For this review, use the dimensioned drawing (mm, ordinates from the lowest corner) and the shaded views. A direction names the side the tool comes from. Give positions to 0.01 mm unless a question says otherwise; leave off trailing zeros. Loops run counter-clockwise (first coordinate to the right, second up) from the corner with the lowest first, then second, coordinate; pieces in that order, holes last. Notation, with made-up numbers: (51.25, -22.5) - (106.25, -22.5) arc R28 cw to (106.25, -1.5) - close; hole circle Ø5 at (79, -31.5). An arc over 180 degrees is marked (long way). Write each question's results on one line, items separated by ' | '.
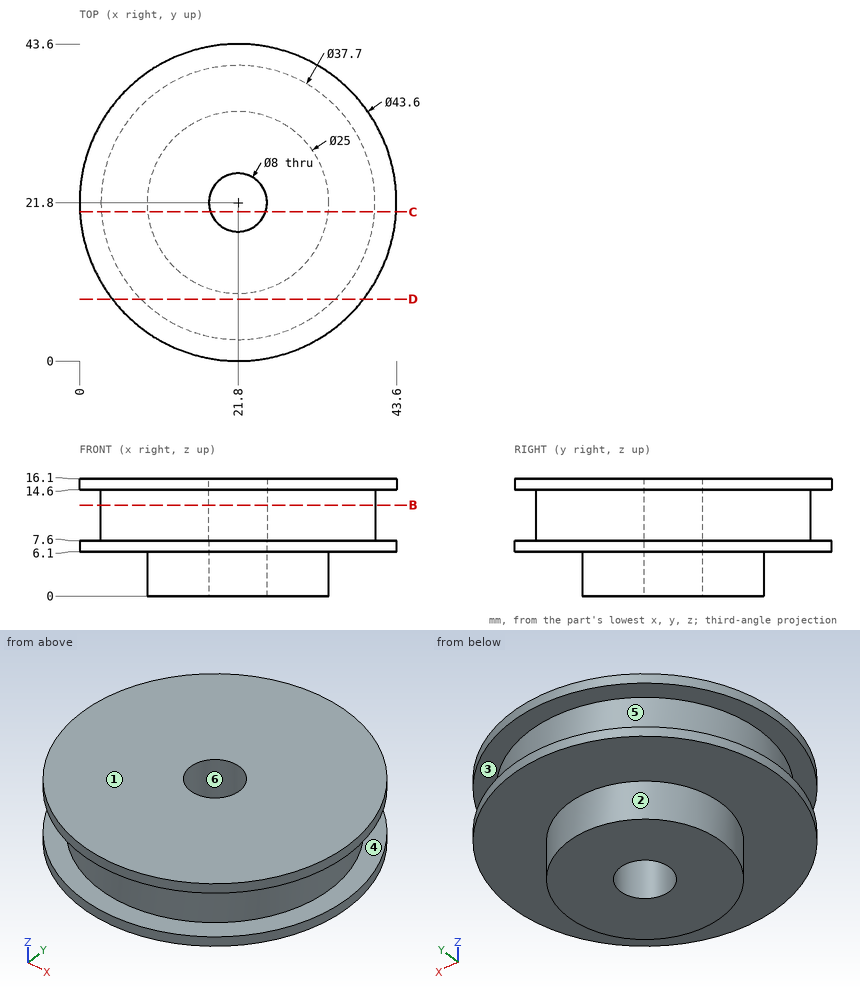
Item 1: We need section B-B on z = 12.5. Give the boundary of the cut face in (x, y), then the cut area to 3 significant figures.
Output values:
outline: circle Ø37.7 at (21.8, 21.8); hole circle Ø8 at (21.8, 21.8) | area: 1,070 mm²
Item 2: Clearance check with flat-ended pins moving along their axes: P1, Ø4, axis at x = 18, z = 14.5, coming from the +Y side; P2, Ø4, axis at x = 13.5, z = 8, coming from the -Y side; P3, Ø6.5, axis at x = 21.8, y = 21.8, coming from the -Z side; P4, Ø6, axis at x = 22, z = 2.5, coming from the +Y side. State where each tip first meets the part, or that it passes through.
Output values:
P1: stops at y = 43.53 | P2: stops at y = 0.94 | P3: passes through | P4: stops at y = 34.3
Item 3: We need section D-D on y = 8.5. Give the boundary of the cut face in (x, z), then the cut area to 3 significant figures.
Output values:
outline: (4.53, 6.1) - (39.07, 6.1) - (39.07, 7.6) - (35.16, 7.6) - (35.16, 14.6) - (39.07, 14.6) - (39.07, 16.1) - (4.53, 16.1) - (4.53, 14.6) - (8.44, 14.6) - (8.44, 7.6) - (4.53, 7.6) - close | area: 291 mm²
Item 4: Tool access review of the marked faces 1, 2 and 3: name each direction out of +Z, -Z, +X, -X, +Y, -Y from which nothing blocks a thin tool from reaching the whole face with its end or side.
Output values:
face 1: +Z, +X, -X, +Y, -Y | face 2: -Z | face 3: none
Item 5: Wall thickness on probe 1 along X at (y, z) = (21.8, 12); probe 2 along Z at (x, y) = (10, 6.5): over which ranges is each line inside the solid? List them lowest first.
Output values:
probe 1: x = 2.95 to 17.8, 25.8 to 40.65 | probe 2: z = 6.1 to 7.6, 14.6 to 16.1
Item 6: Draft analysis for pull direction X (two halves, no side actions). For the marked faces 4, 5 and 6, state which applies: +X half, -X half, draft (parallel to the pull), parting line (faces both ways), or undercut.
Output values:
face 4: draft | face 5: parting line | face 6: undercut
Item 7: We need section C-C on y = 20.5. Give the boundary of the cut face in (x, z), then the cut area to 3 significant figures.
Output values:
outline: (0.04, 6.1) - (9.37, 6.1) - (9.37, 0) - (18.02, 0) - (18.02, 16.1) - (0.04, 16.1) - (0.04, 14.6) - (2.99, 14.6) - (2.99, 7.6) - (0.04, 7.6) - close; (25.58, 0) - (34.23, 0) - (34.23, 6.1) - (43.56, 6.1) - (43.56, 7.6) - (40.61, 7.6) - (40.61, 14.6) - (43.56, 14.6) - (43.56, 16.1) - (25.58, 16.1) - close | area: 424 mm²
